Study the drawing (mm; zero at the part's minimum x, y, z) and answer. A direction names the side the tool comes from. Give positions to 0.01 mm unless a question says otherwise; leave off trailing zeros. Order: outer loops, then holes, each group sorted by start corner. A loop starts at its lowest first (then second) coordinate and runs counter-clockwise, first axis right, second up.
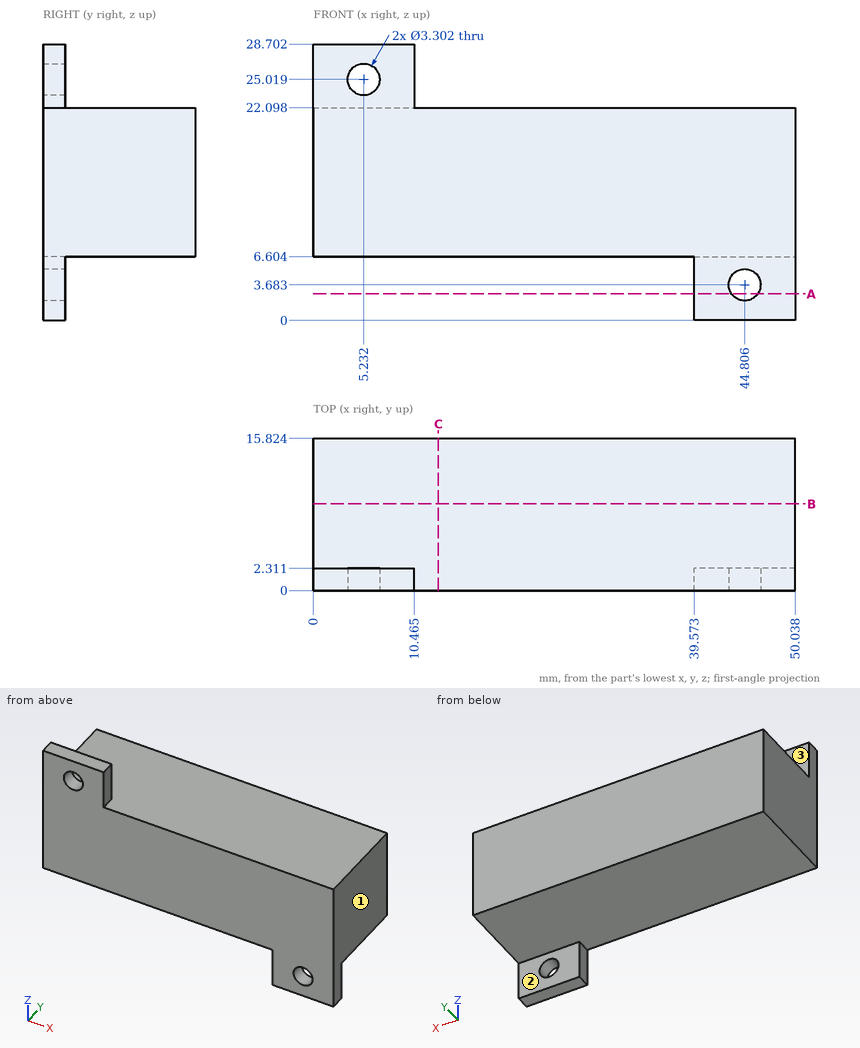
1) Find section C-C (x = 13). Write down the section's boundary in (y, z) (1 decimal), then the cut area to 3 significant figures.
Geometry says:
outline: (0, 6.6) - (15.8, 6.6) - (15.8, 22.1) - (0, 22.1) - close
area: 245 mm2
2) A tool of negligible diameter and unlimited length cuts with its end or side. For the marked faces 1, 2 and 3, from which of +Z, -Z, +X, -X, +Y, -Y can it reach the whole face along a straight path? Write none if from no direction.
Geometry says:
face 1: +Z, -Z, +X, +Y, -Y
face 2: -Z, +X, -X, +Y
face 3: +Z, +X, -X, +Y
3) A straight line is drawn through the part: probe 1 along Z at (x, y) = (41, 5.25). Find the intervals that lie inside material, in ascending order.
Geometry says:
probe 1: z = 6.6 to 22.1
4) Find section A-A (z = 2.75). Write down the section's boundary in (x, y).
Geometry says:
outline: (39.57, 0) - (43.44, 0) - (43.44, 2.31) - (39.57, 2.31) - close; (46.17, 0) - (50.04, 0) - (50.04, 2.31) - (46.17, 2.31) - close
5) Given P1, Ø3.5, axis at x = 45.5, z = 2.5, coming from the +Y side; P2, Ø1, axis at x = 40.5, y = 5, coming from the +Z side; P3, Ø1.8, axis at y = 1, z = 4.5, coming from the -X side, each flat-ended and moving along its own axis, determine where each tip first touches the part or whether it passes through.
Geometry says:
P1: stops at y = 2.31
P2: stops at z = 22.1
P3: stops at x = 39.57
6) Find section B-B (y = 9). Write down the section's boundary in (x, z).
Geometry says:
outline: (0, 6.6) - (50.04, 6.6) - (50.04, 22.1) - (0, 22.1) - close
